Verification items for the finished model (mm, model axes). A direction names the side the tool comes from. Give positions to 0.01 mm unless a question says otherwise; leave off trailing zeros. Loops run counter-clockwise (first coordinate to the right, second up) from the corner with the lowest first, then second, coordinate; pieces in that order, holes last. Notation, with made-up numbers: (82, 86.25) - (90, 86.25) arc R20 cw to (90, 124.25) - close; hole circle Ø1 at (-18.75, -1.75). An arc over 180 degrees is marked (long way). Answer in a Markdown table with one row per item.
```python
from build123d import *

# Parameters (mm, degrees)
BOX067_W          = 12
BOX067_H          = 12
BOX067_DEPTH      = 4
BOX069_W          = 18
BOX069_H          = 8
BOX069_DEPTH      = 3
FILLET031_R       = 3
BOX068_W          = 18
BOX068_H          = 8
BOX068_DEPTH      = 3
FILLET032_R       = 3
BOX066_W          = 12
BOX066_H          = 12
BOX066_DEPTH      = 4
CYLINDER053_R     = 1
CYLINDER053_DEPTH = 8
CYLINDER063_R     = 1
CYLINDER063_DEPTH = 8
CYLINDER060_R     = 1
CYLINDER060_DEPTH = 8
CYLINDER050_R     = 1
CYLINDER050_DEPTH = 8
BOX007_W          = 40
BOX007_H          = 40
BOX007_DEPTH      = 3
CHAMFER009_SIZE   = 2.99
BOX065_W          = 90
BOX065_H          = 90
BOX065_DEPTH      = 66
BOX063_W          = 82
BOX063_H          = 82
BOX063_DEPTH      = 75
FILLET030_R       = 6
BOX064_W          = 90
BOX064_H          = 90
BOX064_DEPTH      = 87
FILLET028_R       = 7


with BuildPart() as cube044:
    # Box067 → Box067 (new body)
    with BuildSketch(Plane(origin=(54, 8, 80), x_dir=(1, 0, 0), z_dir=(0, 0, 1))):
        with Locations((6, 6)):
            Rectangle(BOX067_W, BOX067_H)
    extrude(amount=BOX067_DEPTH)


with BuildPart() as fillet031:
    # Box069 → Box069 (new body)
    with BuildSketch(Plane(origin=(21, 10, 84), x_dir=(1, 0, 0), z_dir=(0, 0, 1))):
        with Locations((9, 4)):
            Rectangle(BOX069_W, BOX069_H)
    extrude(amount=BOX069_DEPTH)

    # Fillet031
    fillet031_edges = [fillet031.edges().sort_by_distance(p)[0] for p in [
        (21, 10, 85.5),
        (21, 18, 85.5),
        (39, 10, 85.5),
        (39, 18, 85.5),
    ]]
    fillet(fillet031_edges, radius=FILLET031_R)


with BuildPart() as fillet032:
    # Box068 → Box068 (new body)
    with BuildSketch(Plane(origin=(51, 10, 84), x_dir=(1, 0, 0), z_dir=(0, 0, 1))):
        with Locations((9, 4)):
            Rectangle(BOX068_W, BOX068_H)
    extrude(amount=BOX068_DEPTH)

    # Fillet032
    fillet032_edges = [fillet032.edges().sort_by_distance(p)[0] for p in [
        (51, 10, 85.5),
        (51, 18, 85.5),
        (69, 10, 85.5),
        (69, 18, 85.5),
    ]]
    fillet(fillet032_edges, radius=FILLET032_R)


with BuildPart() as fusion006:
    # Box066 → Box066 (new body)
    with BuildSketch(Plane(origin=(24, 8, 80), x_dir=(1, 0, 0), z_dir=(0, 0, 1))):
        with Locations((6, 6)):
            Rectangle(BOX066_W, BOX066_H)
    extrude(amount=BOX066_DEPTH)

    # Fusion006: union Cube044, Fillet031, Fillet032
    add(cube044.part)
    add(fillet031.part)
    add(fillet032.part)


with BuildPart() as cylinder058:
    # Cylinder053 → Cylinder053 (new body)
    with BuildSketch(Plane(origin=(9, 9, 78), x_dir=(1, 0, 0), z_dir=(0, 0, 1))):
        Circle(CYLINDER053_R)
    extrude(amount=CYLINDER053_DEPTH)


with BuildPart() as cylinder060:
    # Cylinder063 → Cylinder063 (new body)
    with BuildSketch(Plane(origin=(81, 81, 78), x_dir=(1, 0, 0), z_dir=(0, 0, 1))):
        Circle(CYLINDER063_R)
    extrude(amount=CYLINDER063_DEPTH)


with BuildPart() as cylinder064:
    # Cylinder060 → Cylinder060 (new body)
    with BuildSketch(Plane(origin=(81, 9, 78), x_dir=(1, 0, 0), z_dir=(0, 0, 1))):
        Circle(CYLINDER060_R)
    extrude(amount=CYLINDER060_DEPTH)


with BuildPart() as fusion005:
    # Cylinder050 → Cylinder050 (new body)
    with BuildSketch(Plane(origin=(9, 81, 78), x_dir=(1, 0, 0), z_dir=(0, 0, 1))):
        Circle(CYLINDER050_R)
    extrude(amount=CYLINDER050_DEPTH)

    # Fusion005: union Cylinder058, Cylinder060, Cylinder064
    add(cylinder058.part)
    add(cylinder060.part)
    add(cylinder064.part)


with BuildPart() as chamfer009:
    # Box007 → Box007 (new body)
    with BuildSketch(Plane(origin=(25, 25, 84), x_dir=(1, 0, 0), z_dir=(0, 0, 1))):
        with Locations((20, 20)):
            Rectangle(BOX007_W, BOX007_H)
    extrude(amount=BOX007_DEPTH)

    # Chamfer009
    chamfer009_edges = [chamfer009.edges().sort_by_distance(p)[0] for p in [
        (25, 45, 84),
        (65, 45, 84),
        (45, 25, 84),
        (45, 65, 84),
    ]]
    chamfer(chamfer009_edges, length=CHAMFER009_SIZE)


with BuildPart() as cube042:
    # Box065 → Box065 (new body)
    with BuildSketch(Plane.XY.offset(80)):
        with Locations((45, 45)):
            Rectangle(BOX065_W, BOX065_H)
    extrude(amount=BOX065_DEPTH)


with BuildPart() as fillet030:
    # Box063 → Box063 (new body)
    with BuildSketch(Plane.XY):
        with Locations((41, 41)):
            Rectangle(BOX063_W, BOX063_H)
    extrude(amount=BOX063_DEPTH)

    # Fillet030
    fillet030_edges = [fillet030.edges().sort_by_distance(p)[0] for p in [
        (0, 0, 37.5),
        (0, 41, 75),
        (0, 82, 37.5),
        (82, 0, 37.5),
        (82, 41, 75),
        (82, 82, 37.5),
        (41, 0, 75),
        (41, 82, 75),
    ]]
    fillet(fillet030_edges, radius=FILLET030_R)


with BuildPart() as fillet030_1:
    # Fillet030 placement: moved
    add(fillet030.part.moved(Location((4, 4, 4))))


with BuildPart() as top001:
    # Box064 → Box064 (new body)
    with BuildSketch(Plane.XY):
        with Locations((45, 45)):
            Rectangle(BOX064_W, BOX064_H)
    extrude(amount=BOX064_DEPTH)

    # Fillet028
    fillet028_edges = [top001.edges().sort_by_distance(p)[0] for p in [
        (0, 0, 43.5),
        (0, 45, 87),
        (0, 90, 43.5),
        (90, 0, 43.5),
        (90, 45, 87),
        (90, 90, 43.5),
        (45, 0, 87),
        (45, 90, 87),
    ]]
    fillet(fillet028_edges, radius=FILLET028_R)

    # Cut069: cut Fillet030
    add(fillet030_1.part, mode=Mode.SUBTRACT)

    # Common002: intersect Cube042
    add(cube042.part, mode=Mode.INTERSECT)

    # Cut070: cut Chamfer009
    add(chamfer009.part, mode=Mode.SUBTRACT)

    # Cut071: cut Fusion005
    add(fusion005.part, mode=Mode.SUBTRACT)

    # Cut072: cut Fusion006
    add(fusion006.part, mode=Mode.SUBTRACT)


with BuildPart() as top001_1:
    # Cut072 placement: moved
    add(top001.part.moved(Location((0, 0, 20))))


solid = top001_1.part
```
Q1. Sectioned sample at B-B (z = 102.5). Record the cut outline in (x, y), and give its area (3 significant figures).
Completed:
| item | result |
|---|---|
| outline | (0.46, 7) arc R6.54 ccw to (7, 0.46) - (83, 0.46) arc R6.54 ccw to (89.54, 7) - (89.54, 83) arc R6.54 ccw to (83, 89.54) - (7, 89.54) arc R6.54 ccw to (0.46, 83) - close; hole circle Ø2 at (9, 9); hole circle Ø2 at (9, 81); hole (24, 8) - (36, 8) - (36, 20) - (24, 20) - close; hole (54, 8) - (66, 8) - (66, 20) - (54, 20) - close; hole circle Ø2 at (81, 9); hole circle Ø2 at (81, 81) |
| area | 7,600 mm^2 |
Q2. Go/stop test with flat-tipped pins: P1, Ø1.5, axis at x = 28.5, z = 105, coming from the -Y side; P2, Ø1.2, axis at y = 14.5, z = 102.5, coming from the -X side; P3, Ø1, axis at y = 14, z = 105, coming from the -X side; P4, Ø1.6, axis at x = 30, y = 8.5, coming from the -Z side. Record where each tip stops, or that it passes through.
Completed:
| item | result |
|---|---|
| P1 | y = 1.44 |
| P2 | x = 0.26 |
| P3 | x = 1.64 |
| P4 | z = 100 |
Q3. Tool access check on faces 1 (the face through (54, 14, 102)), 2 (the face through (38.1, 10.86, 105.52)), 3 (the face through (30, 18, 105)). Record the directions out of +Z, -Z, +X, -X, +Y, -Y that give a thin tool (end or side, any length) a straight path to the whole face; none if there is none.
Completed:
| item | result |
|---|---|
| face 1 | -Z |
| face 2 | +Z |
| face 3 | +Z, -Z |
Q4. Thickness scan on line 1 (Y direction, x = 81, z = 103); line 2 (Y direction, x = 81, z = 102.35); line 3 (X direction, y = 9, z = 103.7). Record the ranges inside material, lowest first.
Completed:
| item | result |
|---|---|
| line 1 | 0.68 to 8, 10 to 80, 82 to 89.32 |
| line 2 | 0.41 to 8, 10 to 80, 82 to 89.59 |
| line 3 | 1.06 to 8, 10 to 24, 36 to 54, 66 to 80, 82 to 88.94 |
